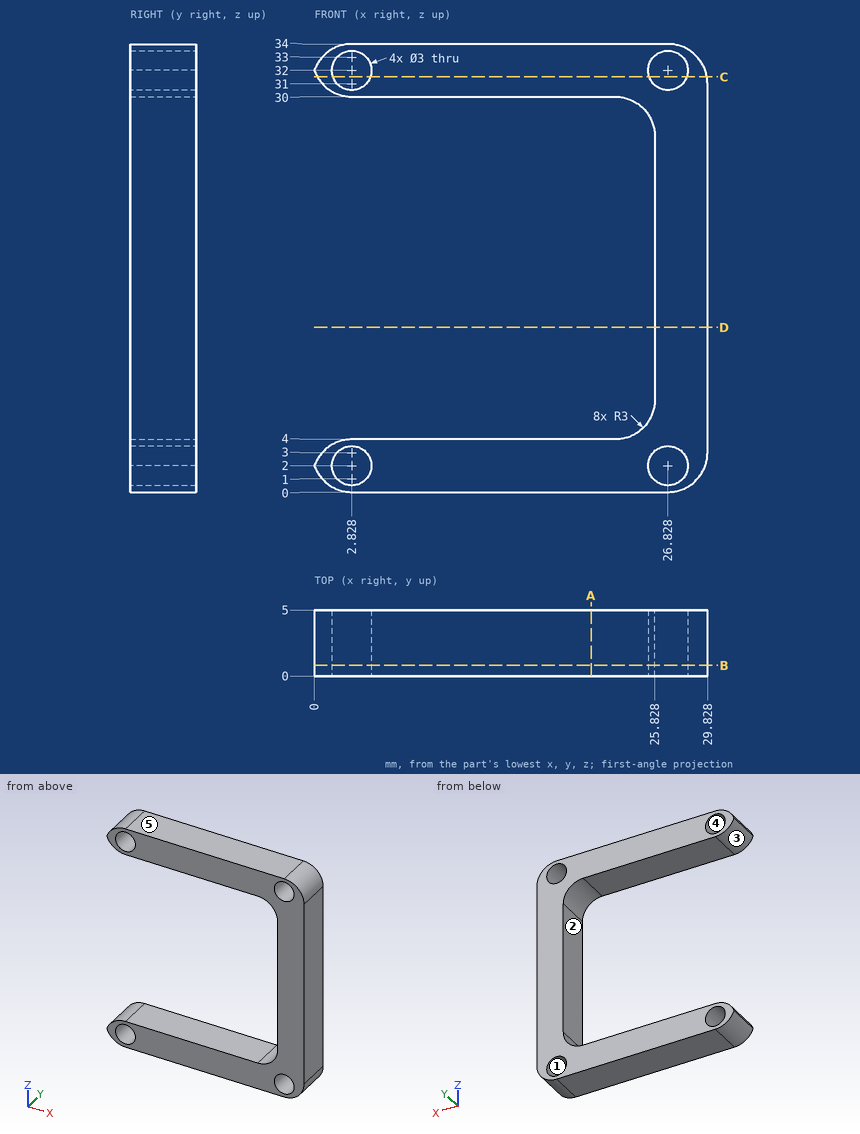
Could you check a few things on this drawing? It's one solid part, dimensions in mm from its lowest x, y, z. A direction names the side the tool comes from. Round coordinates to 2 decimals unless told otherwise and drop trailing zeros. Loops run counter-clockwise (first coordinate to the right, second up) from the corner with the lowest first, then second, coordinate; pieces in that order, holes last.
Q1. I want a section at C-C (z = 31.5). Write out the boundary of the cut face in (x, y) (1 decimal).
Q2. I want a section at A-A (x = 21). Write out the boundary of the cut face in (y, z).
Q3. I want a section at B-B (y = 0.8). Write out the boundary of the cut face in (x, z), and give its area (3 significant figures).
Q4. Thinking about a two-plate mould opening in X: for the marked faces 3, 4 and 5, which applies, pulls with the +X half, pulls with the -X half, needs draft (parallel to the pull), parting line crosses it, or undercut?
Q5. Please list where these lines run through material, in increasing order: L1, parallel to Z at x = 19.25, y = 2.4; L2, parallel to X at y = 2.5, z = 2; L3, parallel to X at y = 1.1, z = 31 (1 decimal).
Q6. On a 3-axis mill with a long thin cutter (end or side, diameter ignored), from which of +Z, -Z, +X, -X, +Y, -Y can I reach the whole of each face in a straight line? I mean the marked faces 1 and 2. Say none if no direction works.
Q7. For P1, Ø3, axis at y = 3, z = 23, coming from the -X side, with a flat end and sliding along its axis, tell me the tip position at first contact or that it passes through.
Q8. I want a section at D-D (z = 12.5). Write out the boundary of the cut face in (x, y).
Answer below:
1. outline: (0.2, 0) - (1.4, 0) - (1.4, 5) - (0.2, 5) - close; (4.2, 0) - (25.4, 0) - (25.4, 5) - (4.2, 5) - close; (28.2, 0) - (29.8, 0) - (29.8, 5) - (28.2, 5) - close
2. outline: (0, 0) - (5, 0) - (5, 4) - (0, 4) - close; (0, 30) - (5, 30) - (5, 34) - (0, 34) - close
3. outline: (0, 2) arc R3 ccw to (2.83, 0) - (26.83, 0) arc R3 ccw to (29.83, 3) - (29.83, 31) arc R3 ccw to (26.83, 34) - (2.83, 34) arc R3 ccw to (0, 32) arc R3 ccw to (2.83, 30) - (22.83, 30) arc R3 cw to (25.83, 27) - (25.83, 7) arc R3 cw to (22.83, 4) - (2.83, 4) arc R3 ccw to start; hole circle Ø3 at (2.83, 2); hole circle Ø3 at (2.83, 32); hole circle Ø3 at (26.83, 2); hole circle Ø3 at (26.83, 32)
3. area: 308 mm2
4. face 3: pulls with the -X half
4. face 4: undercut
4. face 5: needs draft
5. L1: z = 0 to 4, 30 to 34
5. L2: x = 0 to 1.33, 4.33 to 25.33, 28.33 to 29.66
5. L3: x = 0.6 to 1.7, 3.9 to 25.7, 27.9 to 29.8
6. face 1: +Y, -Y
6. face 2: -X, +Y, -Y
7. P1: stops at x = 25.83
8. outline: (25.83, 0) - (29.83, 0) - (29.83, 5) - (25.83, 5) - close
